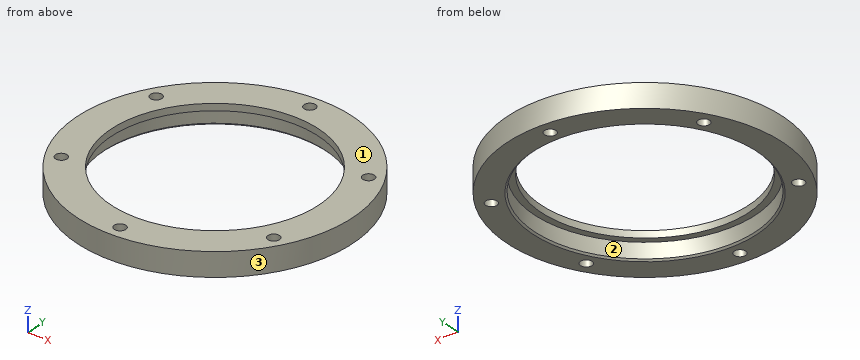
Autodesk Inventor part; units mm, degrees
ref_plane "YZ Plane" through (0, 0, 0) normal (1, 0, 0) x (0, 1, 0)
ref_plane "XZ Plane" through (0, 0, 0) normal (0, 1, 0) x (-1, 0, 0)
ref_plane "XY Plane" through (0, 0, 0) normal (0, 0, 1) x (1, 0, 0)
sketch "スケッチ1" plane through (0, 0, 0) normal (1, 0, 0) x (0, 1, 0)
  line L0 (32.5, 0) -> (32.5, 5)
  line L1 (32.5, 5) -> (30.5, 5)
  line L2 (30.5, 5) -> (30.5, 7)
  line L3 (30.5, 7) -> (40.5, 7)
  line L4 (40.5, 7) -> (40.5, 0)
  line L5 (40.5, 0) -> (32.5, 0)
  line L6 (0, -1.4) -> (0, 8.4)
  point P0 (0, 0)
  dimension "d0" = 32.5
  dimension "d1" = 5
  dimension "d2" = 2
  dimension "d3" = 2
  dimension "d22" = 8
revolve "回転1" add sketch "スケッチ1" angle 360 about axis through (0, 0, -10) along (0, 0, 1)
sketch "スケッチ2" plane through (0, 0, 7) normal (0, 0, 1) x (1, 0, 0)
  circle A0 centre (0, 0) radius 36.5
  point P0 (0, 36.5)
  point P1 (-31.6099, 18.25)
  point P2 (-31.6099, -18.25)
  point P3 (0, -36.5)
  point P4 (31.6099, -18.25)
  point P5 (31.6099, 18.25)
  dimension "d6" = 73
  dimension "d16" = 360
hole "穴1" at (31.6099, 18.25, 7) at (31.6099, -18.25, 7) at (0, -36.5, 7) at (-31.6099, -18.25, 7) at (-31.6099, 18.25, 7) at (0, 36.5, 7) direction (0, 0, -1) diameter 3.4 end through all
chamfer "面取り1" distance 0.5 angle 45 1 edges at (0, -32.5, 0)
properties part number "base2" material "ABS プラスチック"
Part model, mm, in its own coordinate system. Face numbers are marked on the shaded views. Coordinates: 2 decimals unless noted, no trailing zeros. Write each loop counter-clockwise with the first axis right and the second up, starting at its lowest first coordinate (ties: lowest second). Pieces come first, ordered by that corner, then holes.
Item 1: Probe line 1 (Y direction, x = 0, z = 6.1); line 2 (Y direction, x = 0, z = 2.9); line 3 (X direction, y = 0, z = 1.8). List the from-to ranges inside material, lowest first.
Item 2: Slice it at B-B (y = 0). Write the cut outline in (x, z), and give its area (3 significant figures).
Item 3: Slice it at A-A (x = 0). Write the cut outline in (y, z).
Item 4: Pin check, flat tips, straight feed: pin 1 (4 mm diameter, centred on y = 26.5, z = 1, fed in from +X); pin 2 (1 mm diameter, centred on y = -25.5, z = 2.5, fed in from -X); pin 3 (1 mm diameter, centred on y = -25, z = 1, fed in from -X). Stop position of each tip, or through.
Item 5: Slice it at C-C (z = 2.75). Write the cut outline in (x, y), and give its area (3 significant figures).
Item 6: Mould opens along X. For the marked faces 1, 2 and 3 say: released by +X, released by -X, zero draft, split by the parting line, or undercut.
Item 7: Slice it at D-D (y = -17.5). Count the separate pieces of the cut face and the enclosed holes in it, and give its area (3 significant figures).
Results found:
1. line 1: y = -40.5 to -38.2, -34.8 to -30.5, 30.5 to 34.8, 38.2 to 40.5
1. line 2: y = -40.5 to -38.2, -34.8 to -32.5, 32.5 to 34.8, 38.2 to 40.5
1. line 3: x = -40.5 to -32.5, 32.5 to 40.5
2. outline: (-40.5, 0) - (-33, 0) - (-32.5, 0.5) - (-32.5, 5) - (-30.5, 5) - (-30.5, 7) - (-40.5, 7) - close; (30.5, 5) - (32.5, 5) - (32.5, 0.5) - (33, 0) - (40.5, 0) - (40.5, 7) - (30.5, 7) - close
2. area: 120 mm2
3. outline: (-40.5, 0) - (-38.2, 0) - (-38.2, 7) - (-40.5, 7) - close; (-34.8, 0) - (-33, 0) - (-32.5, 0.5) - (-32.5, 5) - (-30.5, 5) - (-30.5, 7) - (-34.8, 7) - close; (30.5, 5) - (32.5, 5) - (32.5, 0.5) - (33, 0) - (34.8, 0) - (34.8, 7) - (30.5, 7) - close; (38.2, 0) - (40.5, 0) - (40.5, 7) - (38.2, 7) - close
4. pin 1: stops at x = 32.25
4. pin 2: stops at x = -31.86
4. pin 3: stops at x = -32.25
5. outline: circle Ø81 at (0, 0); hole circle Ø3.4 at (-31.61, -18.25); hole circle Ø3.4 at (-31.61, 18.25); hole circle Ø65 at (0, 0); hole circle Ø3.4 at (0, -36.5); hole circle Ø3.4 at (0, 36.5); hole circle Ø3.4 at (31.61, -18.25); hole circle Ø3.4 at (31.61, 18.25)
5. area: 1,780 mm2
6. face 1: zero draft
6. face 2: undercut
6. face 3: split by the parting line
7. separate pieces: 4
7. enclosed holes: 0
7. area: 94.5 mm2
